Source: CAD feature listing. Evaluate the final solid. Frame: model axes, mm. A direction names the side the tool comes from. Coordinates: 2 decimals unless noted, no trailing zeros. Order: outer loops, then holes, each group sorted by start corner. A loop starts at its lowest first (then second) coordinate and runs counter-clockwise, first axis right, second up.
Item 1: Section A-A on x = 0. Return the cut outline in (y, z).
Item 2: Reachability of faces 5 (the flat face through (12, 36, -25)), 6 (the cylindrical face through (6.521, 11.352, -3.526)), 7 (the flat face through (13, 36, 25)), 8 (the cylindrical face through (10.3, 2.96, 46.37)), 9 (the flat face through (13, 35, 10)) from +Z, -Z, +X, -X, +Y, -Y: full face, straight path, thin tool, end or side. Return the list, or none.
Item 3: Section B-B on z = 0. Return the cut outline in (x, y), then the cut area to 3 significant figures.
Item 4: Section D-D on z = -22. Return the cut outline in (x, y), then the cut area to 3 significant figures.
Item 5: Section C-C on y = 26. Return the cut outline in (x, z).
Item 6: Mould query, pull axis Y, two halves, no side actions, for faces 1 (the flat face through (12, 66, 0)), 2 (the flat face through (1, 0, 1)), 3 (the cylindrical face through (-0.325, 3.042, 8.464)), 4 (the flat face through (6, 27, 0)). Classes: released by +Y, released by -Y, zero draft, split by the parting line, or undercut.
Item 7: Ray query, line 1 (Z direction, x = 6.75, y = 10); line 2 (Y direction, x = 7.2, z = 5); line 3 (Z direction, x = 6.6, y = 46). Return the intervals inside material, ascending.
Item 8: Contact query for flat-ended pins moving along their axis: P1, Ø1.5, axis at x = 13.5, y = 18.5, coming from the -Z side; P2, Ø6, axis at y = 48.5, z = 6, coming from the +X side; P3, Ø16, axis at y = 29, z = -3, coming from the +X side; P4, Ø15.5, axis at x = 15.5, y = 41.5, coming from the +Z side. Output: stop coordinate, or through.
Autodesk Inventor part; units mm, degrees
ref_plane "YZ Plane" through (0, 0, 0) normal (1, 0, 0) x (0, 1, 0)
ref_plane "XZ Plane" through (0, 0, 0) normal (0, 1, 0) x (-1, 0, 0)
ref_plane "XY Plane" through (0, 0, 0) normal (0, 0, 1) x (1, 0, 0)
sketch "Sketch1" plane through (0, 0, 0) normal (0, 1, 0) x (-1, 0, 0)
  circle A0 centre (0, 0) radius 47.5
  dimension "d0" = 95
extrude "Extrusion1" add sketch "Sketch1" along normal blind 6
sketch "Sketch2" plane through (0, 6, 0) normal (0, 1, 0) x (1, 0, 0)
  circle A0 centre (0, 0) radius 7
  circle A1 centre (0, -7) radius 1.5
  circle A2 centre (0, 7) radius 1.5
  dimension "d3" = 14
  dimension "d4" = 3
  dimension "d5" = 3
extrude "Extrusion2" cut sketch "Sketch2" against normal blind 6 contours A2 A0 | A0 A2 | A1 A0 | A0 A1
sketch "Sketch3" plane through (0, 6, 0) normal (0, 1, 0) x (1, 0, 0)
  line L0 (0, 0) -> (5, 0)
  line L1 (5, 0) -> (5, -10)
  line L2 (5, -10) -> (0, -10)
  line L3 (0, -10) -> (0, 0)
  line L4 (5, 0) -> (0, 0)
  line L5 (0, 0) -> (0, 10)
  line L6 (0, 10) -> (5, 10)
  line L7 (5, 10) -> (5, 0)
  line L8 (5, 0) -> (20, 0)
  line L9 (20, 0) -> (20, -25)
  line L10 (20, -25) -> (5, -25)
  line L11 (5, -25) -> (5, 0)
  line L12 (20, 0) -> (5, 0)
  line L13 (5, 0) -> (5, 25)
  line L14 (5, 25) -> (20, 25)
  line L15 (20, 25) -> (20, 0)
  dimension "d8" = 5
  dimension "d9" = 10
  dimension "d10" = 10
  dimension "d11" = 15
  dimension "d12" = 25
  dimension "d13" = 25
extrude "Extrusion3" add sketch "Sketch3" along normal blind 60 contours L8 L9 L10 L11 L1 | L7 L13 L14 L15 L8
sketch "Sketch4" plane through (5, 6, -25) normal (-1, 0, 0) x (0, 0, 1)
  line L0 (50, 0) -> (50, 60)
  line L1 (50, 0) -> (48, 0)
  line L2 (48, 0) -> (48, 40)
  line L3 (48, 40) -> (50, 40)
  line L4 (50, 40) -> (50, 0)
  circle A0 centre (25, 40) radius 10
  point P0 (25, -6)
  dimension "d16" = 2
  dimension "d17" = 40
  dimension "d18" = 20
extrude "Extrusion4" cut sketch "Sketch4" against normal blind 20 contours A0
sketch "Sketch5" plane through (20, 6, 25) normal (1, 0, 0) x (0, 0, -1)
  circle A0 centre (25, 40) radius 10
  line L0 (25, 40) -> (30, 40)
  line L1 (30, 40) -> (30, 4)
  line L2 (30, 4) -> (25, 4)
  line L3 (25, 4) -> (25, 40)
  line L4 (25, 40) -> (20, 40)
  line L5 (20, 40) -> (20, 4)
  line L6 (20, 4) -> (25, 4)
  line L7 (25, 4) -> (25, 40)
  circle A1 centre (20, 4) radius 2
  circle A2 centre (30, 4) radius 2
  point P0 (25, -6)
  dimension "d21" = 5
  dimension "d22" = 36
  dimension "d23" = 5
  dimension "d24" = 36
  dimension "d25" = 4
  dimension "d26" = 4
extrude "Extrusion5" cut sketch "Sketch5" against normal blind 20 contours A1 L6 L5 | L5 L6 A1 | A2 L2 L1 | L1 L2 A2
sketch "Sketch6" plane through (20, 6, 25) normal (1, 0, 0) x (0, 0, -1)
  line L0 (25, 40) -> (30, 40)
  line L1 (30, 40) -> (30, 54)
  line L2 (30, 54) -> (25, 54)
  line L3 (25, 54) -> (25, 40)
  line L4 (25, 40) -> (20, 40)
  line L5 (20, 40) -> (20, 54)
  line L6 (20, 54) -> (25, 54)
  line L7 (25, 54) -> (25, 40)
  circle A0 centre (20, 54) radius 2
  circle A1 centre (30, 54) radius 2
  point P0 (25, -6)
  dimension "d29" = 5
  dimension "d30" = 14
  dimension "d31" = 5
  dimension "d32" = 14
  dimension "d33" = 4
  dimension "d34" = 4
extrude "Extrusion6" cut sketch "Sketch6" against normal blind 20 contours A1 L2 L1 | L1 L2 A1 | A0 L5 L6 | L6 L5 A0
sketch "Sketch7" plane through (20, 6, 25) normal (1, 0, 0) x (0, 0, -1)
  line L0 (20, 54) -> (30, 54)
  line L1 (30, 54) -> (30, 4)
  line L2 (30, 4) -> (20, 4)
  line L3 (20, 4) -> (20, 54)
  circle A0 centre (20, 54) radius 2
  line L4 (0, 0) -> (0, 60)
  line L5 (20, 54) -> (0, 54)
  line L6 (0, 54) -> (0, 49)
  line L7 (0, 49) -> (20, 49)
  line L8 (20, 49) -> (20, 54)
  circle A1 centre (25, 40) radius 10
  line L9 (25, 40) -> (15, 40)
  line L10 (15, 40) -> (15, 30)
  line L11 (15, 30) -> (25, 30)
  line L12 (25, 30) -> (25, 40)
  line L13 (25, 40) -> (35, 40)
  line L14 (35, 40) -> (35, 30)
  line L15 (35, 30) -> (25, 30)
  line L16 (25, 30) -> (25, 40)
  line L17 (35, 40) -> (15, 40)
  line L18 (15, 40) -> (15, 9)
  line L19 (15, 9) -> (35, 9)
  line L20 (35, 9) -> (35, 40)
  line L21 (15, 9) -> (35, 9)
  line L22 (35, 9) -> (35, 49)
  line L23 (35, 49) -> (15, 49)
  line L24 (15, 49) -> (15, 9)
  point P0 (25, -6)
  point P1 (30, 49)
  point P2 (30, 48.6603)
  point P3 (15, 49)
  point P4 (20, 48.6603)
  dimension "d37" = 10
  dimension "d38" = 50
  dimension "d39" = 5
  dimension "d40" = 10
  dimension "d41" = 10
  dimension "d42" = 10
  dimension "d43" = 31
  dimension "d44" = 40
extrude "Extrusion7" cut sketch "Sketch7" against normal blind 14 contours L3 A1 L24 L7 | L23 L22 A1 L1 | A1 L3 L11 L10 | L14 L15 L1 A1 | A1 L11 L3 | L11 L3 L19 L18 | L1 L15 A1 | L20 L19 L1 L15 | L11 L15 L1 L19 L3
sketch "Sketch8" plane through (20, 6, 25) normal (1, 0, 0) x (0, 0, -1)
  line L0 (15, 40) -> (15, 49)
  line L1 (15, 49) -> (35, 49)
  line L2 (35, 49) -> (35, 56)
  line L3 (35, 56) -> (15, 56)
  line L4 (15, 56) -> (15, 49)
  line L5 (35, 9) -> (15, 9)
  line L6 (15, 9) -> (35, 9)
  line L7 (35, 9) -> (35, 2)
  line L8 (35, 2) -> (15, 2)
  line L9 (15, 2) -> (15, 9)
  point P0 (25, -6)
  dimension "d47" = 20
  dimension "d48" = 7
  dimension "d49" = 20
  dimension "d50" = 7
sketch "Sketch9" plane through (20, 6, 25) normal (1, 0, 0) x (0, 0, -1)
  line L0 (15, 40) -> (15, 49)
  circle A0 centre (25, 40) radius 10
  line L1 (15, 49) -> (35, 49)
  line L2 (35, 49) -> (35, 40)
  line L3 (35, 40) -> (15, 40)
  line L4 (15, 40) -> (15, 49)
  line L5 (15, 49) -> (20, 49)
  line L6 (20, 49) -> (20.777, 49)
  line L7 (20.777, 49) -> (20.777, 48.469)
  line L8 (20.777, 48.469) -> (20, 48.469)
  line L9 (20, 48.469) -> (20, 49)
  line L10 (30, 49) -> (35, 49)
  line L11 (30, 49) -> (29.2041, 49)
  line L12 (29.2041, 49) -> (29.2041, 48.469)
  line L13 (29.2041, 48.469) -> (30, 48.469)
  line L14 (30, 48.469) -> (30, 49)
  line L15 (35, 49) -> (35, 9)
  line L16 (15, 56) -> (35, 56)
  line L17 (35, 56) -> (35, 49)
  line L18 (35, 49) -> (15, 49)
  line L19 (15, 49) -> (15, 56)
  line L20 (15, 9) -> (15, 49)
  line L21 (15, 9) -> (35, 9)
  line L22 (35, 9) -> (35, 2)
  line L23 (35, 2) -> (15, 2)
  line L24 (15, 2) -> (15, 9)
  point P0 (25, -6)
  point P1 (20, 48.6603)
  point P2 (30, 48.6603)
  dimension "d51" = 7
extrude "Extrusion8" cut sketch "Sketch9" against normal blind 12 contours L19 L16 L17 L1 A0 | L9 L1 A0 | L21 L22 L23 L24 | A0 L1 L14
sketch "Sketch10" plane through (8, 60, -5) normal (1, 0, 0) x (0, 0, -1)
  line L0 (-10, -5) -> (-10, -5.3397)
  line L1 (-10, -5) -> (0, -5)
  line L2 (0, -5) -> (0, -5.5581)
  line L3 (0, -5.5581) -> (-10, -5.5581)
  line L4 (-10, -5.5581) -> (-10, -5)
  point P0 (-5, -60)
extrude "Extrusion9" cut sketch "Sketch10" against normal blind 2
properties part number "BaseTop"
Answer list:
1. outline: (0, -47.5) - (6, -47.5) - (6, -8.5) - (0, -8.5) - close; (0, -5.5) - (6, -5.5) - (6, 5.5) - (0, 5.5) - close; (0, 8.5) - (6, 8.5) - (6, 47.5) - (0, 47.5) - close
2. face 5: -Z, +X, -X, +Y
2. face 6: +X, -X
2. face 7: +Z, +X, -X, +Y
2. face 8: +Y, -Y
2. face 9: +X
3. outline: (-47.5, 0) - (47.5, 0) - (47.5, 6) - (20, 6) - (20, 8) - (8, 8) - (8, 15) - (6, 15) - (6, 36) - (5, 36) - (5, 6) - (-47.5, 6) - close; (5, 56) - (8, 56) - (8, 62) - (20, 62) - (20, 66) - (5, 66) - close
3. area: 720 mm2
4. outline: (-42.1, 0) - (42.1, 0) - (42.1, 6) - (20, 6) - (20, 66) - (5, 66) - (5, 6) - (-42.1, 6) - close
4. area: 1,410 mm2
5. outline: (5, -25) - (20, -25) - (20, -10) - (6, -10) - (6, 10) - (20, 10) - (20, 25) - (5, 25) - close
6. face 1: released by +Y
6. face 2: released by -Y
6. face 3: zero draft
6. face 4: undercut
7. line 1: z = -25 to -7, -3 to 3, 7 to 25
7. line 2: y = 0 to 8, 12 to 15, 55 to 58, 62 to 66
7. line 3: z = -25 to -10, 10 to 25
8. P1: stops at z = -25
8. P2: passes through
8. P3: stops at x = 20
8. P4: stops at z = 25
